Geometry: final body of the model. Coordinates: model frame, mm. Face numbers are marked on the shaded views. Round coordinates to 2 decimals unless told otherwise and drop trailing zeros. Write each loop counter-clockwise with the first axis right and the second up, starting at its lowest first coordinate (ties: lowest second). Pieces come first, ordered by that corner, then holes. Notation, with made-up numbers: (36, 46) - (63, 46) arc R17 cw to (63, 69) - close; hole circle Ø9 at (70, -33). An arc over 180 degrees is marked (long way). Write each question's results on one line, items separated by ' | '.
Solid Edge part; units mm, degrees
sketch "Sketch1" plane through (0, 0, 0) normal (0, 0, 1) x (1, 0, 0)
  line L0 (-33.2164, -43.334) -> (33.2164, -43.334)
  arc A0 (33.2164, -43.334) -> (-33.2164, -43.334) centre (0, 0) ccw
extrude "Protrusion1" add sketch "Sketch1" against normal blind 0.4
sketch "Sketch2" plane through (0, 9.1432, 0) normal (0, 0, 1) x (-1, 0, 0)
  line L0 (-35, 57.8772) -> (35, 57.8772)
  arc A0 (-35, 57.8772) -> (35, 57.8772) centre (0, 9.1432) ccw
extrude "Protrusion2" add sketch "Sketch2" along normal blind 2
sketch "Sketch3" plane through (0, 8.1307, 2) normal (0, 0, 1) x (1, 0, 0)
  line L0 (-7.3, 27.3693) -> (7.3, 27.3693)
  line L1 (7.3, 27.3693) -> (7.3, 0.105)
  arc A0 (-7.3, 0.105) -> (7.3, 0.105) centre (0, -8.1307) ccw
  line L2 (-7.3, 27.3693) -> (-7.3, 0.105)
  circle A1 centre (10.25, 0.1693) radius 0.95
  circle A2 centre (10.25, 20.8693) radius 0.95
  circle A3 centre (-10.25, 20.8693) radius 0.95
  circle A4 centre (-10.25, 0.1693) radius 0.95
extrude "Cutout1" cut sketch "Sketch3" against normal through all
hole "Hole1" at (29.7724, 29.7694, 2) direction (0, 0, -1) diameter 3.4 end up to next
pattern_circular "Pattern1" count 6 over 360 about axis through (0, 0, 2) along (0, 0, -1) of "Hole1"
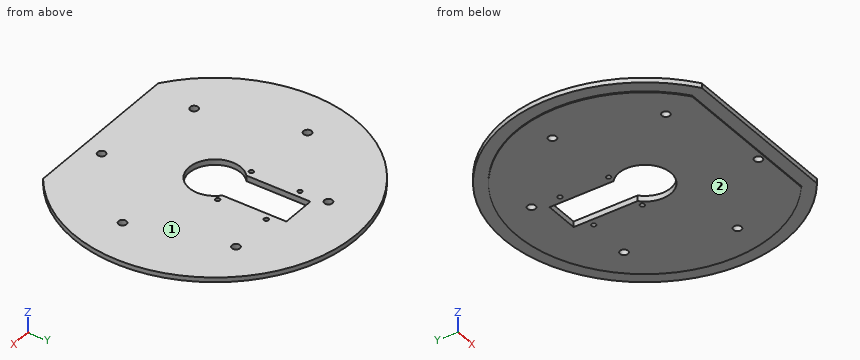
Q1. Pin query (flat end, axial travel): pin 1 (1 mm diameter, centred on y = -0.5, z = 0, fed in from -X). Return the tip coordinate at first contact, or that it passes through.
Answer block:
pin 1: x = -60
Q2. Section query C-C, the plane z = 1.5. Give the number of separate pieces and of enclosed holes in the cut face, plus the area to 3 significant figures.
Answer block:
separate pieces: 1 | enclosed holes: 11 | area: 9,960 mm2
Q3. Section query A-A, the plane x = 0. Return loops of the section in (y, z).
Answer block:
outline: (-48.73, 0) - (-43.33, 0) - (-43.33, -0.4) - (-11.01, -0.4) - (-11.01, 2) - (-48.73, 2) - close; (35.5, -0.4) - (54.6, -0.4) - (54.6, 0) - (60, 0) - (60, 2) - (35.5, 2) - close
Q4. Section query D-D, the plane y = 37. Return loops of the section in (x, z).
Answer block:
outline: (-47.23, 0) - (-40.15, 0) - (-40.15, -0.4) - (40.15, -0.4) - (40.15, 0) - (47.23, 0) - (47.23, 2) - (-47.23, 2) - close
Q5. Section query B-B, the plane y = 0. Return loops of the section in (x, z), plus the area to 3 significant figures.
Answer block:
outline: (-60, 0) - (-54.6, 0) - (-54.6, -0.4) - (-11.01, -0.4) - (-11.01, 2) - (-60, 2) - close; (11.01, -0.4) - (54.6, -0.4) - (54.6, 0) - (60, 0) - (60, 2) - (11.01, 2) - close | area: 231 mm2
Q6. Ray query, line 1 along X through (y, z) = (7.5, 1.35); line 2 along X through (y, z) = (10.5, 0.9); line 3 along X through (y, z) = (5.5, 1.35). Return the intervals inside material, ascending.
Answer block:
line 1: -59.53 to -10.76, -9.74 to -8.05, 8.05 to 9.74, 10.76 to 59.53 | line 2: -59.07 to -42.32, -39.01 to -7.3, 7.3 to 59.07 | line 3: -59.75 to -9.53, 9.53 to 59.75
Q7. Mould query, pull axis Z, two halves, no side actions, for the marked faces 1 and 2. Classes: pulls with the +Z half, pulls with the -Z half, needs draft (parallel to the pull), parting line crosses it, or undercut.
Answer block:
face 1: pulls with the +Z half | face 2: pulls with the -Z half
